from build123d import *

# Parameters (mm, degrees)
F0_W     = 99.370434
F0_H     = 41.450106
F1_DEPTH = 127
F2_R     = 14.029552
F3_DEPTH = 127.001
F4_R     = 3.175


with BuildPart() as f1:
    # F0 (on Front) → F1 (new body)
    with BuildSketch(Plane.XZ):
        Rectangle(F0_W, F0_H)
    extrude(amount=-F1_DEPTH)

    # F2 (on face) → F3 (cut, through all)
    with BuildSketch(Plane.XZ):
        Circle(F2_R)
    extrude(amount=-F3_DEPTH, mode=Mode.SUBTRACT)

    # F4
    f4_edges = [f1.edges().sort_by_distance(p)[0] for p in [
        (49.685217, 63.5, 20.725053),
        (-49.685217, 63.5, 20.725053),
        (0, 0, 20.725053),
        (0, 127, 20.725053),
    ]]
    fillet(f4_edges, radius=F4_R)


solid = f1.part
Work out the finished part from the listing and answer in its coordinate system (mm). Round coordinates to 2 decimals unless told otherwise and drop trailing zeros. Loops run counter-clockwise (first coordinate to the right, second up) from the corner with the lowest first, then second, coordinate; pieces in that order, holes last. Notation, with made-up numbers: (-31.5, 59.25) -> (-22.5, 59.25) arc R15 cw to (-22.5, 84.25) -> close; hole circle Ø2 at (58, -9). An arc over 180 degrees is marked (long way). Use one line per item in the form item = value.
(1) Find section A-A on y = 95. Give the vertices of the cut face in (x, z) (3 decimals), then the cut area to 3 significant figures.
Answer list:
outline = (-49.685, -20.725) -> (49.685, -20.725) -> (49.685, 17.55) arc R3.175 ccw to (46.51, 20.725) -> (-46.51, 20.725) arc R3.175 ccw to (-49.685, 17.55) -> close; hole circle Ø28.059 at (0, 0)
area = 3,500 mm2
(2) Find section D-D on z = -9.5. Give the vertices of the cut face in (x, y).
Answer list:
outline = (-49.69, 0) -> (-10.32, 0) -> (-10.32, 127) -> (-49.69, 127) -> close; (10.32, 0) -> (49.69, 0) -> (49.69, 127) -> (10.32, 127) -> close
(3) Find section C-C on x = 0. Give the vertices of the cut face in (y, z) (3 decimals).
Answer list:
outline = (0, -20.725) -> (127, -20.725) -> (127, -14.03) -> (0, -14.03) -> close; (0, 14.03) -> (127, 14.03) -> (127, 17.55) arc R3.175 ccw to (123.825, 20.725) -> (3.175, 20.725) arc R3.175 ccw to (0, 17.55) -> close
(4) Straight lines are drawn through the part: line 1 (Z direction, x = 0, y = 31); line 2 (Z direction, x = 5, y = 102); line 3 (X direction, y = 44, z = -12). For each, find the intervals that lie inside material, in ascending order.
Answer list:
line_1 = -20.73 to -14.03, 14.03 to 20.73
line_2 = -20.73 to -13.11, 13.11 to 20.73
line_3 = -49.69 to -7.27, 7.27 to 49.69
(5) Find section B-B on z = 0. Give the vertices of the cut face in (x, y), then the cut area to 3 significant figures.
Answer list:
outline = (-49.69, 0) -> (-14.03, 0) -> (-14.03, 127) -> (-49.69, 127) -> close; (14.03, 0) -> (49.69, 0) -> (49.69, 127) -> (14.03, 127) -> close
area = 9,060 mm2
(6) A flat-ended cylindrical pin translates along its axis: P1, Ø10, axis at x = -37.5, z = 6.5, coming from the -Y side. Find the tip coordinate at first contact, or state that the pin passes through.
Answer list:
P1 = 0
(7) For a pull along Z with two mould halves and no side action, classify faces 1 (the cylindrical face through (-10.34, 62.61, 9.48)), 2 (the cylindrical face through (-48.78, 64.39, 19.77)), 3 (the flat face through (49.685, 63, -2)) as released by +Z, released by -Z, zero draft, split by the parting line, or undercut.
Answer list:
face_1 = undercut
face_2 = released by +Z
face_3 = zero draft
